Geometry: final body of the model. Coordinates: model frame, mm. Face numbers are marked on the shaded views. A direction names the side the tool comes from. Round coordinates to 2 decimals unless told otherwise and drop trailing zeros. Order: outer loops, then holes, each group sorted by start corner. A loop starts at its lowest first (then second) coordinate and runs counter-clockwise, first axis right, second up. Notation, with made-up numbers: (19.25, 49) - (70.25, 49) arc R19 ccw to (70.25, 81) - close; hole circle Ø9 at (-36, 83.5). An arc over 180 degrees is marked (long way). Put each result on its own line as item: value. Start each with the question number.
(1) Section B-B (x = 0). Output: boundary loops of the cut face in (y, z).
(2) Section C-C (y = 4). Output: boundary loops of the cut face in (x, z).
(3) Pin query (flat end, axial travel): P1, Ø4, axis at x = 16.5, y = 10, coming from the +Z side; P2, Ø2, axis at y = 6.5, z = -1.5, coming from the +X side; P3, Ø1.5, axis at y = 15.5, z = -5, coming from the +X side; P4, Ø0.6, axis at x = -0.5, z = -1, coming from the -Y side. Return the tip coordinate at first contact, or that it passes through.
(4) Access query for the marked faces 3 and 4. Directions: +Z, -Z, +X, -X, +Y, -Y. A direction counts if a zero-diameter tool reaches every point of the face in a straight line with its end or side. Return the directions, or none.
(5) Pull-direction query (X, two-part tool) for the marked faces 1 and 2; classes: released by +X, released by -X, zero draft, split by the parting line, or undercut.
(6) Section A-A (z = -4.25). Output: boundary loops of the cut face in (x, y), and give its area (3 significant figures).
(7) Material intervals for L1, parallel to X at y = -13, z = -0.5; L2, parallel to X at y = 0, z = -2.9; L3, parallel to Z at x = 4, y = -11, sorted ascending. Write a range as [from, to].
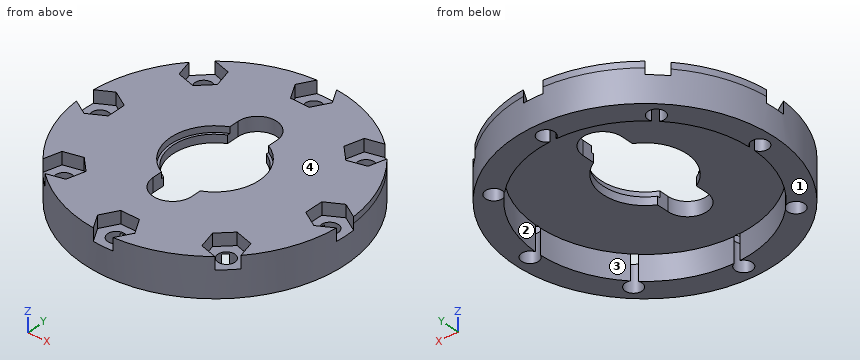
from build123d import *

# Parameters (mm, degrees)
SKETCH3_R           = 21
BOSS_EXTRUDE2_DEPTH = 1
SKETCH4_R           = 21
BOSS_EXTRUDE3_DEPTH = 5.28
SKETCH5_R           = 17.25
CUT_EXTRUDE1_DEPTH  = 4
CUT_EXTRUDE2_DEPTH  = 2
SKETCH8_R           = 1.35
CUT_EXTRUDE4_DEPTH  = 7.28
CIRPATTERN1_COUNT   = 8
CUT_EXTRUDE5_DEPTH  = 7.28


with BuildPart() as part:
    # Sketch3 → Boss-Extrude2 (new body)
    with BuildSketch(Plane.XY):
        Circle(SKETCH3_R)
        with BuildLine():
            Line((-3.124988, -6.403130094), (-3.124988, -7.949679))
            Line((-3.124988, -7.949679), (3.125012, -7.949679))
            Line((3.125012, -7.949679), (3.125012, -6.403118381))
            ThreePointArc((3.125012, -6.403118381), (7.125, 0), (3.125012, 6.403118381))
            Line((3.125012, 6.403118381), (3.125012, 7.949431))
            Line((3.125012, 7.949431), (-3.124988, 7.949431))
            Line((-3.124988, 7.949431), (-3.124988, 6.403130094))
            ThreePointArc((-3.124988, 6.403130094), (-7.125, 0), (-3.124988, -6.403130094))
        make_face(mode=Mode.SUBTRACT)
    extrude(amount=-BOSS_EXTRUDE2_DEPTH)

    # Sketch4 → Boss-Extrude3 (add)
    with BuildSketch(Plane(origin=(0, 0, -1), x_dir=(-1, 0, 0), z_dir=(0, 0, -1))):
        Circle(SKETCH4_R)
        with BuildLine():
            Line((2.749988, 6.164419356), (2.749988, 7.574431))
            Line((2.749988, 7.574431), (-2.750012, 7.574431))
            Line((-2.750012, 7.574431), (-2.750012, 6.16440865))
            ThreePointArc((-2.750012, 6.16440865), (-6.75, 0), (-2.750012, -6.16440865))
            Line((-2.750012, -6.16440865), (-2.750012, -7.574679))
            Line((-2.750012, -7.574679), (2.749988, -7.574679))
            Line((2.749988, -7.574679), (2.749988, -6.164419356))
            ThreePointArc((2.749988, -6.164419356), (6.75, 0), (2.749988, 6.164419356))
        make_face(mode=Mode.SUBTRACT)
    extrude(amount=BOSS_EXTRUDE3_DEPTH)

    # Sketch5 → Cut-Extrude1 (cut)
    with BuildSketch(Plane(origin=(0, 0, -6.28), x_dir=(-1, 0, 0), z_dir=(0, 0, -1))):
        Circle(SKETCH5_R)
    extrude(amount=-CUT_EXTRUDE1_DEPTH, mode=Mode.SUBTRACT)

    # Sketch6 → Cut-Extrude2 (cut)
    with BuildSketch(Plane.XY):
        Polygon((-21.1, -1.5011107), (-18.5, -3.0022214), (-15.9, -1.5011107), (-15.9, 1.5011107), (-18.5, 3.0022214), (-21.1, 1.5011107), align=None)
    cut_extrude2 = extrude(amount=-CUT_EXTRUDE2_DEPTH, mode=Mode.SUBTRACT)

    # Sketch8 → Cut-Extrude4 (cut, through all)
    with BuildSketch(Plane.XY):
        with Locations((-18.5, 0)):
            Circle(SKETCH8_R)
    cut_extrude4 = extrude(amount=-CUT_EXTRUDE4_DEPTH, mode=Mode.SUBTRACT)

    # CirPattern1: Cut-Extrude2, Cut-Extrude4 ×8 about axis
    cirpattern1_axis = Axis((0, 0, 0), (0, 0, 1))
    for i in range(1, CIRPATTERN1_COUNT):
        add(cut_extrude2.rotate(cirpattern1_axis, i * 360 / CIRPATTERN1_COUNT), mode=Mode.SUBTRACT)
        add(cut_extrude4.rotate(cirpattern1_axis, i * 360 / CIRPATTERN1_COUNT), mode=Mode.SUBTRACT)

    # Sketch9 → Cut-Extrude5 (cut, through all)
    with BuildSketch(Plane.XY):
        with BuildLine():
            Line((3.125012, 7.949431), (3.125012, -7.949431))
            ThreePointArc((3.125012, -7.949431), (1.2e-05, -11.074431), (-3.124988, -7.949431))
            Line((-3.124988, -7.949431), (-3.124988, 7.949431))
            ThreePointArc((-3.124988, 7.949431), (1.2e-05, 11.074431), (3.125012, 7.949431))
        make_face()
    extrude(amount=-CUT_EXTRUDE5_DEPTH, mode=Mode.SUBTRACT)


solid = part.part
Checks:
1. outline: (-21, -6.28) - (-19.85, -6.28) - (-19.85, -2) - (-21, -2) - close; (-17.15, -2.28) - (-11.07, -2.28) - (-11.07, 0) - (-15.9, 0) - (-15.9, -2) - (-17.15, -2) - close; (11.07, -2.28) - (17.15, -2.28) - (17.15, -2) - (15.9, -2) - (15.9, 0) - (11.07, 0) - close; (19.85, -6.28) - (21, -6.28) - (21, -2) - (19.85, -2) - close
2. outline: (-20.62, -6.28) - (-16.78, -6.28) - (-16.78, -2.28) - (-5.44, -2.28) - (-5.44, -1) - (-5.9, -1) - (-5.9, 0) - (-20.62, 0) - close; (5.44, -2.28) - (16.78, -2.28) - (16.78, -6.28) - (20.62, -6.28) - (20.62, 0) - (5.9, 0) - (5.9, -1) - (5.44, -1) - close
3. P1: stops at z = 0
3. P2: stops at x = 20.27
3. P3: stops at x = 14.95
3. P4: stops at y = -15.9
4. face 3: -Z
4. face 4: +Z, +X, -X, +Y, -Y
5. face 1: zero draft
5. face 2: undercut
6. outline: circle Ø42 at (0, 0); hole (-17.24, -0.49) arc R17.25 ccw to (-12.54, -11.84) arc R1.35 ccw (long way) to (-11.84, -12.54) arc R17.25 ccw to (-0.49, -17.24) arc R1.35 ccw (long way) to (0.49, -17.24) arc R17.25 ccw to (11.84, -12.54) arc R1.35 ccw (long way) to (12.54, -11.84) arc R17.25 ccw to (17.24, -0.49) arc R1.35 ccw (long way) to (17.24, 0.49) arc R17.25 ccw to (12.54, 11.84) arc R1.35 ccw (long way) to (11.84, 12.54) arc R17.25 ccw to (0.49, 17.24) arc R1.35 ccw (long way) to (-0.49, 17.24) arc R17.25 ccw to (-11.84, 12.54) arc R1.35 ccw (long way) to (-12.54, 11.84) arc R17.25 ccw to (-17.24, 0.49) arc R1.35 ccw (long way) to start
6. area: 405 mm²
7. L1: x = [-16.49, -15.75], [-10.37, 10.37], [15.75, 16.49]
7. L2: x = [-21, -19.85], [19.85, 21]
7. L3: z = [-2.28, 0]
